The model under review builds one solid part; all positions refer to its coordinate system, in mm. A direction names the side the tool comes from. Give positions to 0.01 mm unless a question says otherwise; leave off trailing zeros. Order: outer loops, then holes, each group sorted by start corner. A loop starts at its lowest first (then second) coordinate and runs counter-clockwise, first axis right, second up.
```python
from build123d import *

# Parameters (mm, degrees)
SKETCH1_R           = 3
BOSS_EXTRUDE1_DEPTH = 2.5
SKETCH2_W           = 9
SKETCH2_H           = 4.761904762
BOSS_EXTRUDE2_DEPTH = 5
FILLET1_R           = 2
CHAMFER1_SIZE       = 1
FILLET2_R           = 1
SKETCH3_R           = 1.5
CUT_EXTRUDE1_DEPTH  = 20


with BuildPart() as part:
    # Sketch1 → Boss-Extrude1 (new body, symmetric)
    with BuildSketch(Plane.XY):
        with BuildLine():
            Line((0, 10), (-20, 10))
            Line((-20, 10), (-20, 0))
            Line((-20, 0), (-14, 0))
            Line((-14, 0), (-10, -4))
            Line((-10, -4), (-10, -10))
            Line((-10, -10), (0, -10))
            ThreePointArc((0, -10), (10, 0), (0, 10))
        make_face()
        Circle(SKETCH1_R, mode=Mode.SUBTRACT)
    extrude(amount=BOSS_EXTRUDE1_DEPTH, both=True)

    # Sketch2 → Boss-Extrude2 (add, symmetric)
    with BuildSketch(Plane.XY):
        with Locations((-15.5, 7.619047619)):
            Rectangle(SKETCH2_W, SKETCH2_H)
    extrude(amount=BOSS_EXTRUDE2_DEPTH, both=True)

    # Fillet1
    fillet1_edges = [part.edges().sort_by_distance(p)[0] for p in [
        (-15.5, 10, -5),
        (-15.5, 10, 5),
    ]]
    fillet(fillet1_edges, radius=FILLET1_R)

    # Chamfer1
    chamfer1_edges = [part.edges().sort_by_distance(p)[0] for p in [
        (-3, 0, -2.5),
        (-3, 0, 2.5),
    ]]
    chamfer(chamfer1_edges, length=CHAMFER1_SIZE)

    # Fillet2
    fillet2_edges = [part.edges().sort_by_distance(p)[0] for p in [
        (-5, -10, 2.5),
        (10, 0, 2.5),
        (-5.5, 10, 2.5),
        (-5.5, 10, -2.5),
        (10, 0, -2.5),
        (-5, -10, -2.5),
    ]]
    fillet(fillet2_edges, radius=FILLET2_R)

    # Sketch3 → Cut-Extrude1 (cut)
    with BuildSketch(Plane(origin=(0, 10, 0), x_dir=(1, 0, 0), z_dir=(0, 1, 0))):
        with Locations((-15, 0)):
            Circle(SKETCH3_R)
    extrude(amount=-CUT_EXTRUDE1_DEPTH, mode=Mode.SUBTRACT)


solid = part.part
```
1. Take a section at A-A (z = 0). Write out the cut boundary in (x, y), and give its area (3 significant figures).
2. Insertion check: pin 1 (8 mm diameter, centred on x = -14, y = -3, fed in from -Z); pin 2 (4 mm diameter, centred on y = -5.5, z = -1, fed in from -X); pin 3 (10 mm diameter, centred on x = -11, y = 0, fed in from +Z). Each pin has a flat end and moves straight along its axis. Give the tip position at first contact, or say it passes through.
3. For faces 4 (the flat face through (-16, 7, 5)), 5 (the cylindrical face through (-5.577, 9.715, 2.199)), 6 (the flat face through (-16, 5.238, 4)), 7 (the flat face through (-18, 0, 0)), list the 3-axis set-ups (+Z, -Z, +X, -X, +Y, -Y) from which the entire face can be reached by the end or side of a thin tool; tool diameter is ignored.
4. Take a section at C-C (z = 4.25). Write out the cut boundary in (x, y), and give its area (3 significant figures).
5. To check wall thickness, follow line 1 (Y direction, x = 0, z = 0.1); line 2 (X direction, y = 2.25, z = 0); line 3 (X direction, y = 1.5, z = 0). State the ranges of each line that lie inside material, in increasing order.
6. Take a section at B-B (x = -15). Write out the cut boundary in (y, z).
7. Draft analysis for pull direction X (two halves, no side actions). For faces 1 (the cylindrical face through (-16.5, 4.82, -0.07)), 2 (the flat face through (-5, -10, 0)), 3 (the flat face through (-10, -7, 0)), state which applies: pulls with the +X half, pulls with the -X half, needs draft (parallel to the pull), parting line crosses it, or undercut.
Answer:
1. outline: (-20, 0) - (-16.5, 0) - (-16.5, 10) - (-20, 10) - close; (-13.5, -0.5) - (-10, -4) - (-10, -10) - (0, -10) arc R10 ccw to (0, 10) - (-13.5, 10) - close; hole circle Ø6 at (0, 0)
1. area: 407 mm2
2. pin 1: stops at z = -2.5
2. pin 2: stops at x = -10.5
2. pin 3: stops at z = 2.5
3. face 4: +Z, +X, -X, +Y, -Y
3. face 5: +Z, +X, +Y
3. face 6: +Z, +X, -X, -Y
3. face 7: +Z, -Z, -X, -Y
4. outline: (-20, 5.24) - (-11, 5.24) - (-11, 9.56) - (-20, 9.56) - close
4. area: 38.9 mm2
5. line 1: y = -10 to -3, 3 to 10
5. line 2: x = -20 to -16.5, -13.5 to -1.98, 1.98 to 9.74
5. line 3: x = -20 to -16.5, -13.5 to -2.6, 2.6 to 9.89
6. outline: (0, -2.5) - (5.24, -2.5) - (5.24, -5) - (8, -5) arc R2 ccw to (10, -3) - (10, -1.5) - (0, -1.5) - close; (0, 1.5) - (10, 1.5) - (10, 3) arc R2 ccw to (8, 5) - (5.24, 5) - (5.24, 2.5) - (0, 2.5) - close
7. face 1: undercut
7. face 2: needs draft
7. face 3: pulls with the -X half
